Autodesk Inventor part; units mm, degrees
ref_plane "Work Plane1" through (0, 0, 13.1) normal (0, 0, 1) x (1, 0, 0)
ref_plane "YZ Plane" through (0, 0, 0) normal (1, 0, 0) x (0, 1, 0)
ref_plane "XZ Plane" through (0, 0, 0) normal (0, 1, 0) x (-1, 0, 0)
sketch "Sketch1" plane through (0, 0, 0) normal (0, 0, 1) x (1, 0, 0)
  circle A0 centre (0, 0) radius 17.5
  circle A1 centre (0, 0) radius 8
  circle A2 centre (0, 0) radius 5.5
  circle A3 centre (0, 0) radius 2.75
  circle A4 centre (0, 0) radius 13 construction
  point P0 (0, 13)
  point P1 (-13, 0)
  point P2 (0, -13)
  point P3 (13, 0)
  dimension "d10" = 26
  dimension "d0" = 35
  dimension "d1" = 16
  dimension "d2" = 11
  dimension "d3" = 5.5
  dimension "d13" = 360
extrude "Extrusion1" add sketch "Sketch1" along normal blind 4 contours A0 | A1 | A2
extrude "Extrusion2" add sketch "Sketch1" along normal blind 21 contours A1 | A2
extrude "Extrusion3" cut sketch "Sketch1" along normal blind 16 contours A2
hole "Hole1" at (0, -13, 0) at (13, 0, 0) at (0, 13, 0) at (-13, 0, 0) direction (0, 0, 1) diameter 3.242 end through all
ref_plane "Work Plane1" through (0, 0, 13.1) normal (0, 0, 1) x (1, 0, 0)
sketch "Sketch2" plane through (0, 0, 13.1) normal (0, 0, 1) x (1, 0, 0)
  circle A0 centre (0, 0) radius 6
  dimension "d23" = 12
extrude "Extrusion4" cut sketch "Sketch2" against normal blind 1.1
chamfer "Chamfer1" distance 0.25 angle 45 1 edges at (-8, 0, 21)
chamfer "Chamfer2" distance 0.1 angle 45 6 edges at (-17.5, 0, 4) (-17.5, 0, 0) (-13, -1.621, 0) (0, -14.621, 0) (0, 11.379, 0) (13, -1.621, 0)
properties part number "BearingSuport"
Work out the finished part from the listing and answer in its coordinate system (mm). A direction names the side the tool comes from. Coordinates: 2 decimals unless noted, no trailing zeros. Loops run counter-clockwise (first coordinate to the right, second up) from the corner with the lowest first, then second, coordinate; pieces in that order, holes last. Notation, with made-up numbers: M -36,-34 L 13,-34 A29 ccw 13,-10 Z; hole C 46.25,61.5 d1. An arc over 180 degrees is marked long. Use CSV: the item, a comma, the result in double quotes. Start each with the question number.
(1) Consider line 1 (Y direction, x = 0, z = 2.6); line 2 (Z direction, x = -10, y = 8.5); line 3 (Y direction, x = -13, z = 1.95). Determine where each line is inside the solid, lowest interval first.
(2) Given pin 1 Ø14 at (x, y) = (0, 0) entering from +Z; pin 2 Ø2 at (y, z) = (-5, 17.5) entering from -X; pin 3 Ø5 at (x, z) = (7, 8.5) entering from +Y; pin 4 Ø8 at (x, z) = (5.5, 12.5) entering from -Y, each flat-ended and moving along its own axis, determine where each tip first touches the part or whether it passes through.
(3) Find section A-A, the plane x = 0. State how many separate pieces and enclosed holes the cut face has, then the cut area to 3 significant figures.
(4) Find section B-B, the plane z = 5.25. Give the vertices of the cut face in (x, y).
(5) For faces 1 (the face through (-1.19, 5.37, 14.53)), 2 (the face through (-5.994, 0.264, 12.558)), 3 (the face through (-14.607, -0.211, 2.077)), determine the directions among +Z, -Z, +X, -X, +Y, -Y from which every point of the face is accessible in a straight line to the end or side of a thin tool.
(6) For a pull along Y with two mould halves and no side action, classify faces 4 (the face through (-1.73, 7.81, 12.26)), 5 (the face through (0.621, 14.497, 2.077)), 6 (the face through (0, -3, 21)) as +Y half, -Y half, draft (parallel to the pull), parting line (faces both ways), or undercut.
Recorded:
1,line 1,"y = -17.5 to -14.62, -11.38 to -5.5, 5.5 to 11.38, 14.62 to 17.5"
1,line 2,"z = 0 to 4"
1,line 3,"y = -11.72 to -1.62, 1.62 to 11.72"
2,pin 1,"stops at z = 21"
2,pin 2,"stops at x = -6.93"
2,pin 3,"stops at y = 6.61"
2,pin 4,"stops at y = -7.86"
3,separate pieces,"4"
3,enclosed holes,"0"
3,area,"181 mm^2"
4,outline,"C 0,0 d16; hole C 0,0 d11"
5,face 1,"-Z"
5,face 2,"none"
5,face 3,"+Z, -Z"
6,face 4,"parting line"
6,face 5,"undercut"
6,face 6,"draft"
